```python
from build123d import *

# Parameters (mm, degrees)
SKETCH1_W           = 215
SKETCH1_H           = 90
BOSS_EXTRUDE1_DEPTH = 5
CUT_EXTRUDE2_DEPTH  = 146.187632354
SKETCH7_W           = 90
SKETCH7_H           = 10
BOSS_EXTRUDE3_DEPTH = 70
SKETCH8_W           = 10
SKETCH8_H           = 10
CUT_EXTRUDE4_DEPTH  = 38


with BuildPart() as part:
    # Sketch1 → Boss-Extrude1 (new, symmetric)
    with BuildSketch(Plane(origin=(0, 0, 0), x_dir=(1, 0, 0), z_dir=(0, 1, 0))):
        with Locations((6.317611065, 0.819935691)):
            Rectangle(SKETCH1_W, SKETCH1_H)
    extrude(amount=BOSS_EXTRUDE1_DEPTH, both=True)

    # Sketch3 → Cut-Extrude2 (cut, through all)
    with BuildSketch(Plane.XY.offset(44.180064309)):
        with BuildLine():
            Line((-101.182388935, -5), (-76.182388935, -5))
            Line((-76.182388935, -5), (-76.182388935, -2))
            Line((-76.182388935, -2), (-86.182388935, -1))
            Line((-86.182388935, -1), (-92.067313838, -1))
            ThreePointArc((-92.067313838, -1), (-92.876019978, -1.111056529), (-93.624851386, -1.436003747))
            ThreePointArc((-93.624851386, -1.436003747), (-98.180146552, 1.243963481), (-93.431421846, 3.563996253))
            ThreePointArc((-93.431421846, 3.563996253), (-92.600234286, 3.144478048), (-91.680454758, 3))
            Line((-91.680454758, 3), (-86.182388935, 3))
            Line((-86.182388935, 3), (-76.182388935, 4))
            Line((-76.182388935, 4), (-76.182388935, 5))
            Line((-76.182388935, 5), (-101.182388935, 5))
            Line((-101.182388935, 5), (-101.182388935, -5))
        make_face()
    extrude(amount=-CUT_EXTRUDE2_DEPTH, mode=Mode.SUBTRACT)

    # Sketch7 → Boss-Extrude3 (add)
    with BuildSketch(Plane(origin=(113.817611065, 0, 0), x_dir=(0, 0, -1), z_dir=(1, 0, 0))):
        with Locations((0.819935691, 0)):
            Rectangle(SKETCH7_W, SKETCH7_H)
    extrude(amount=BOSS_EXTRUDE3_DEPTH)

    # Sketch8 → Cut-Extrude4 (cut)
    with BuildSketch(Plane(origin=(0, 5, 0), x_dir=(1, 0, 0), z_dir=(0, 1, 0))):
        with Locations((-24.27998453, -29.180064309)):
            Rectangle(SKETCH8_W, SKETCH8_H)
        with Locations((-56.27998453, -29.180064309)):
            Rectangle(SKETCH8_W, SKETCH8_H)
        with Locations((7.72001547, -29.180064309)):
            Rectangle(SKETCH8_W, SKETCH8_H)
        with Locations((39.72001547, -29.180064309)):
            Rectangle(SKETCH8_W, SKETCH8_H)
        with Locations((71.72001547, -29.180064309)):
            Rectangle(SKETCH8_W, SKETCH8_H)
        with Locations((103.72001547, -29.180064309)):
            Rectangle(SKETCH8_W, SKETCH8_H)
        with Locations((135.72001547, -29.180064309)):
            Rectangle(SKETCH8_W, SKETCH8_H)
        with Locations((-24.27998453, -9.180064309)):
            Rectangle(SKETCH8_W, SKETCH8_H)
        with Locations((7.72001547, -9.180064309)):
            Rectangle(SKETCH8_W, SKETCH8_H)
        with Locations((39.72001547, -9.180064309)):
            Rectangle(SKETCH8_W, SKETCH8_H)
        with Locations((71.72001547, -9.180064309)):
            Rectangle(SKETCH8_W, SKETCH8_H)
        with Locations((103.72001547, -9.180064309)):
            Rectangle(SKETCH8_W, SKETCH8_H)
        with Locations((135.72001547, -9.180064309)):
            Rectangle(SKETCH8_W, SKETCH8_H)
        with Locations((-24.27998453, 10.819935691)):
            Rectangle(SKETCH8_W, SKETCH8_H)
        with Locations((7.72001547, 10.819935691)):
            Rectangle(SKETCH8_W, SKETCH8_H)
        with Locations((39.72001547, 10.819935691)):
            Rectangle(SKETCH8_W, SKETCH8_H)
        with Locations((71.72001547, 10.819935691)):
            Rectangle(SKETCH8_W, SKETCH8_H)
        with Locations((103.72001547, 10.819935691)):
            Rectangle(SKETCH8_W, SKETCH8_H)
        with Locations((135.72001547, 10.819935691)):
            Rectangle(SKETCH8_W, SKETCH8_H)
        with Locations((-24.27998453, 30.819935691)):
            Rectangle(SKETCH8_W, SKETCH8_H)
        with Locations((7.72001547, 30.819935691)):
            Rectangle(SKETCH8_W, SKETCH8_H)
        with Locations((39.72001547, 30.819935691)):
            Rectangle(SKETCH8_W, SKETCH8_H)
        with Locations((71.72001547, 30.819935691)):
            Rectangle(SKETCH8_W, SKETCH8_H)
        with Locations((103.72001547, 30.819935691)):
            Rectangle(SKETCH8_W, SKETCH8_H)
        with Locations((135.72001547, 30.819935691)):
            Rectangle(SKETCH8_W, SKETCH8_H)
        with Locations((-56.27998453, -9.180064309)):
            Rectangle(SKETCH8_W, SKETCH8_H)
        with Locations((-56.27998453, 10.819935691)):
            Rectangle(SKETCH8_W, SKETCH8_H)
        with Locations((-56.27998453, 30.819935691)):
            Rectangle(SKETCH8_W, SKETCH8_H)
    cut_extrude4 = extrude(amount=-CUT_EXTRUDE4_DEPTH, mode=Mode.SUBTRACT)

    # Mirror2: Cut-Extrude4 across plane
    add(cut_extrude4.mirror(Plane.ZY.offset(-150.72001547)), mode=Mode.SUBTRACT)


solid = part.part
```
Build history of the part. All positions in model axes, mm. Give positions to 0.01 mm unless a question says otherwise; leave off trailing zeros. Loops run counter-clockwise (first coordinate to the right, second up) from the corner with the lowest first, then second, coordinate; pieces in that order, holes last.
Item 1: Slice it at B-B, the plane z = -1. List the corners of the cut face in (x, y).
Answers follow:
outline: (-93.62, -1.44) arc R3 cw to (-92.07, -1) - (-86.18, -1) - (-76.18, -2) - (-76.18, -5) - (183.82, -5) - (183.82, 5) - (-76.18, 5) - (-76.18, 4) - (-86.18, 3) - (-91.68, 3) arc R3 cw to (-93.43, 3.56) arc R3 ccw (long way) to start
Item 2: Pull direction Z, two halves, no side cores. Call faces 1 (the face through (72, 0, -5.82)), 2 (the face through (52, -5, 0)): released by +Z, released by -Z, zero draft, split by the parting line, or undercut.
Answers follow:
face 1: undercut
face 2: zero draft
Item 3: Slice it at C-C, the plane y = -3.5. Give the number of separate pieces and of enclosed holes in the cut face, and give its area (3 significant figures).
Answers follow:
separate pieces: 1
enclosed holes: 32
area: 20,200 mm2
Item 4: Drill centre lines: line 1 (Z direction, x = 70.5, y = 0.5); line 2 (X direction, y = -3.25, z = -40); line 3 (X direction, y = 1.5, z = -38.5). Where is each one in solid material? Low to high.
Answers follow:
line 1: z = -45.82 to -35.82, -25.82 to -15.82, -5.82 to 4.18, 14.18 to 24.18, 34.18 to 44.18
line 2: x = -76.18 to 183.82
line 3: x = -98.16 to 183.82
Item 5: Slice it at A-A, the plane x = -56.5. List the corners of the cut face in (y, z), and give its area (3 significant figures).
Answers follow:
outline: (-5, -45.82) - (5, -45.82) - (5, -35.82) - (-5, -35.82) - close; (-5, -25.82) - (5, -25.82) - (5, -15.82) - (-5, -15.82) - close; (-5, -5.82) - (5, -5.82) - (5, 4.18) - (-5, 4.18) - close; (-5, 14.18) - (5, 14.18) - (5, 24.18) - (-5, 24.18) - close; (-5, 34.18) - (5, 34.18) - (5, 44.18) - (-5, 44.18) - close
area: 500 mm2
